The listing builds one solid part. Answer for the finished solid, in the listing's coordinates (mm). Face numbers are marked on the shaded views. A direction names the side the tool comes from. Coordinates: 2 decimals unless noted, no trailing zeros. Loops run counter-clockwise (first coordinate to the right, second up) from the corner with the lowest first, then second, coordinate; pieces in that order, holes last. Notation, with made-up numbers: (79, 7.5) - (112, 7.5) arc R21 ccw to (112, 27.5) - close; hole circle Ø6 at (77, -14). An arc over 180 degrees is marked (long way). Use one line per item in the form item = value. Start each with the question number.
```python
from build123d import *

# Parameters (mm, degrees)
SKETCH035_R          = 1.6
PAD_DEPTH            = 61.5
PAD_DEPTH_BACK       = 61.5
SKETCH038_W          = 14.8
SKETCH038_H          = 8
SKETCH038_W_2        = 59.6
POCKET001_DEPTH      = 4
POCKET001_DEPTH_BACK = 4
SKETCH039_W          = 119
SKETCH039_H          = 67.4
POCKET002_DEPTH      = 11
POCKET003_DEPTH      = 13.001
SKETCH041_W          = 11.6
SKETCH041_H          = 3.5
SKETCH041_W_2        = 14.8
SKETCH041_H_2        = 8
POCKET004_DEPTH      = 2
POCKET005_DEPTH      = 2
POCKET006_DEPTH      = 2
POCKET011_DEPTH      = 3
POCKET012_DEPTH      = 3
SKETCH051_W          = 14.8
SKETCH051_H          = 4
SKETCH051_W_2        = 59.6
POCKET013_DEPTH      = 0.4
CHAMFER_SIZE         = 1


with BuildPart() as part:
    # Sketch035 (on Face1 of Binder) → Pad (new body, two sides)
    with BuildSketch(Plane.YZ) as pad_sk:
        with BuildLine():
            ThreePointArc((4, 0), (-2.828418, 2.828436), (-2.6e-05, -4))
            Line((-2.6e-05, -4), (4.4, -4))
            Line((4.4, -4), (4.4, -13))
            Line((4.4, -13), (75.8, -13))
            Line((75.8, -13), (75.8, 0))
            Line((75.8, 0), (4, 0))
        make_face()
        Circle(SKETCH035_R, mode=Mode.SUBTRACT)
    extrude(amount=PAD_DEPTH)
    extrude(pad_sk.sketch, amount=-PAD_DEPTH_BACK)

    # Sketch038 → Pocket001 (cut, two sides)
    with BuildSketch(Plane.XY) as pocket001_sk:
        with Locations((-54.1, 0)):
            Rectangle(SKETCH038_W, SKETCH038_H)
        Rectangle(SKETCH038_W_2, SKETCH038_H)
        with Locations((54.1, 0)):
            Rectangle(SKETCH038_W, SKETCH038_H)
    extrude(amount=-POCKET001_DEPTH, mode=Mode.SUBTRACT)
    extrude(pocket001_sk.sketch, amount=POCKET001_DEPTH_BACK, mode=Mode.SUBTRACT)

    # Sketch039 → Pocket002 (cut)
    with BuildSketch(Plane.XY):
        with Locations((0, 40.1)):
            Rectangle(SKETCH039_W, SKETCH039_H)
    extrude(amount=-POCKET002_DEPTH, mode=Mode.SUBTRACT)

    # Sketch040 → Pocket003 (cut, through all)
    with BuildSketch(Plane.XY):
        with BuildLine():
            ThreePointArc((-24.1, 70.6), (-27.6, 67.1), (-24.1, 63.6))
            Line((-24.1, 63.6), (-19.6, 63.6))
            ThreePointArc((-19.6, 63.6), (-16.1, 67.1), (-19.6, 70.6))
            Line((-24.1, 70.6), (-19.6, 70.6))
        make_face()
    extrude(amount=-POCKET003_DEPTH, mode=Mode.SUBTRACT)

    # Sketch041 (on Face16 of Pocket003) → Pocket004 (cut)
    with BuildSketch(Plane(origin=(0, 75.8, 0), x_dir=(-1, 0, 0), z_dir=(0, 1, 0))):
        with Locations((-29.3, -6.25)):
            Rectangle(SKETCH041_W, SKETCH041_H)
        with Locations((0.6, -7)):
            Rectangle(SKETCH041_W_2, SKETCH041_H_2)
    extrude(amount=-POCKET004_DEPTH, mode=Mode.SUBTRACT)

    # Sketch042 (on Face9 of Pocket004) → Pocket005 (cut)
    with BuildSketch(Plane.XZ.offset(-4.4)):
        Polygon((22.5, -5), (33.1, -5), (33.1, -11), (31, -11), (31, -13), (24.6, -13), (24.6, -11), (22.5, -11), align=None)
        Polygon((36.9, -5), (36.9, -11), (39, -11), (39, -13), (45.4, -13), (45.4, -11), (47.5, -11), (47.5, -5), align=None)
    extrude(amount=-POCKET005_DEPTH, mode=Mode.SUBTRACT)

    # Sketch043 (on Face10 of Pocket005) → Pocket006 (cut)
    with BuildSketch(Plane.YZ.offset(61.5)):
        Polygon((57.8, -5), (68.4, -5), (68.4, -11), (66.3, -11), (66.3, -13), (59.9, -13), (59.9, -11), (57.8, -11), align=None)
        with BuildLine():
            Line((11.6, -3.5), (21.6, -3.5))
            ThreePointArc((21.6, -10.5), (25.1, -7), (21.6, -3.5))
            Line((21.6, -10.5), (11.6, -10.5))
            ThreePointArc((11.6, -3.5), (8.1, -7), (11.6, -10.5))
        make_face()
    extrude(amount=-POCKET006_DEPTH, mode=Mode.SUBTRACT)

    # Sketch049 (on Face14 of Pocket006) → Pocket011 (cut)
    with BuildSketch(Plane(origin=(29.8, 0, 0), x_dir=(0, -1, 0), z_dir=(-1, 0, 0))):
        Polygon((2.771281, 1.6), (0, 3.2), (-2.771281, 1.6), (-2.771281, -1.6), (0, -3.2), (2.771281, -1.6), align=None)
    extrude(amount=-POCKET011_DEPTH, mode=Mode.SUBTRACT)

    # Sketch050 (on Face4 of Pocket011) → Pocket012 (cut)
    with BuildSketch(Plane.YZ.offset(-29.8)):
        Polygon((2.771281, -1.6), (2.771281, 1.6), (0, 3.2), (-2.771281, 1.6), (-2.771281, -1.6), (0, -3.2), align=None)
    extrude(amount=-POCKET012_DEPTH, mode=Mode.SUBTRACT)

    # Sketch051 (on Face15 of Pocket012) → Pocket013 (cut)
    with BuildSketch(Plane.XZ.offset(-4)):
        with Locations((54.1, -2)):
            Rectangle(SKETCH051_W, SKETCH051_H)
        with Locations((0, -2)):
            Rectangle(SKETCH051_W_2, SKETCH051_H)
        with Locations((-54.1, -2)):
            Rectangle(SKETCH051_W, SKETCH051_H)
    extrude(amount=-POCKET013_DEPTH, mode=Mode.SUBTRACT)

    # Chamfer
    chamfer_edges = [part.edges().sort_by_distance(p)[0] for p in [
        (35.1, 75.8, -6.25),
        (29.3, 75.8, -4.5),
        (23.5, 75.8, -6.25),
        (29.3, 75.8, -8),
        (6.8, 75.8, -7),
        (-8, 75.8, -7),
        (-0.6, 75.8, -3),
        (-0.6, 75.8, -11),
    ]]
    chamfer(chamfer_edges, length=CHAMFER_SIZE)


solid = part.part
```
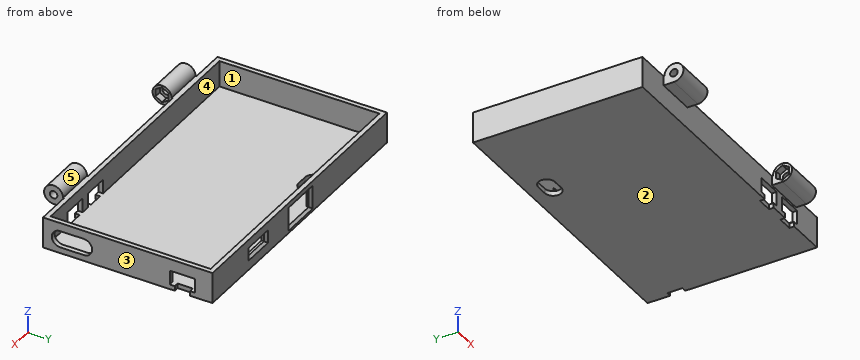
(1) A cutting plane is placed at A-A (x = 43.5). Determine the outline of the cut face in (y, z), then the cut area to 3 significant figures.
(2) A cutting plane is placed at B-B (x = 26). Determine the outline of the cut face in (y, z).
(3) Find the intervals of material crossed by probe 1 along X at (y, z) = (46, -1.75); probe 2 along Z at (x, y) = (36, 0); probe 3 along Y at (x, z) = (14, -0.5), in increasing order. Write a range as from..to.
(4) For the marked faces 1 and 2, determine the directions among +Z, -Z, +X, -X, +Y, -Y from which every point of the face is accessible in a straight line to the end or side of a thin tool.
(5) Determine the mould class of the marked faces 3, 4 and 5 for opening direction Y: +Y half, -Y half, draft (parallel to the pull), parting line (faces both ways), or undercut.
(6) A cutting plane is placed at C-C (y = 42). Determine the outline of the cut face in (x, z).
(7) A cutting plane is placed at D-D (x = -54). Determine the outline of the cut face in (y, z).
(8) Each of these flat-tipped pins is pushed along its axis until it touches: pin 1 Ø1.5 at (x, z) = (-31, 0.5) entering from +Y; pin 2 Ø0.8 at (x, y) = (30, 74.5) entering from +Z; pin 3 Ø2 at (x, y) = (17.5, 21) entering from +Z; pin 4 Ø1 at (y, z) = (63, -12) entering from +X. Where does it stop, or does it pass through?
Evaluation:
q1.outline = (0, -4) - (4.4, -4) - (4.4, -5) - (6.4, -5) - (6.4, 0) - (4, 0) arc R4 ccw (long way) to start; (6.4, -13) - (75.8, -13) - (75.8, 0) - (73.8, 0) - (73.8, -11) - (6.4, -11) - close; hole circle Ø3.2 at (0, 0)
q1.area = 218 mm^2
q2.outline = (4.4, -5) - (6.4, -5) - (6.4, 0) - (4.4, 0) - close; (6.4, -13) - (75.8, -13) - (75.8, -9) - (74.8, -8) - (73.8, -8) - (73.8, -11) - (6.4, -11) - close; (73.8, -4.5) - (74.8, -4.5) - (75.8, -3.5) - (75.8, 0) - (73.8, 0) - close
q3.probe_1 = -61.5..-59.5, 59.5..61.5
q3.probe_2 = -4..-1.6, 1.6..4
q3.probe_3 = 4.4..6.4, 73.8..75.8
q4.face_1 = +Z
q4.face_2 = -Z, +X, -X, +Y, -Y
q5.face_3 = draft
q5.face_4 = undercut
q5.face_5 = parting line
q6.outline = (-61.5, -13) - (61.5, -13) - (61.5, 0) - (59.5, 0) - (59.5, -11) - (-59.5, -11) - (-59.5, 0) - (-61.5, 0) - close
q7.outline = (4.4, -13) - (75.8, -13) - (75.8, 0) - (73.8, 0) - (73.8, -11) - (6.4, -11) - (6.4, 0) - (4.4, 0) - close
q8.pin_1 = 75.8
q8.pin_2 = 0
q8.pin_3 = -11
q8.pin_4 = 59.5
